Geometry: see drawing. Coordinates: mm, zero at the bounding-box minimum. A direction names the side the tool comes from. Give positions to 0.01 mm unless a question says otherwise; leave off trailing zeros. Order: outer loops, then holes, each group sorted by start corner. A loop starts at its lowest first (then second) coordinate and runs counter-clockwise, first axis right, second up. Notation, with made-up numbers: (13.5, 68.25) - (42.5, 68.25) arc R29 cw to (42.5, 100.25) - close; hole circle Ø6 at (-13.75, 35.25). An arc over 180 degrees is marked (long way). One line per item, written item: value.
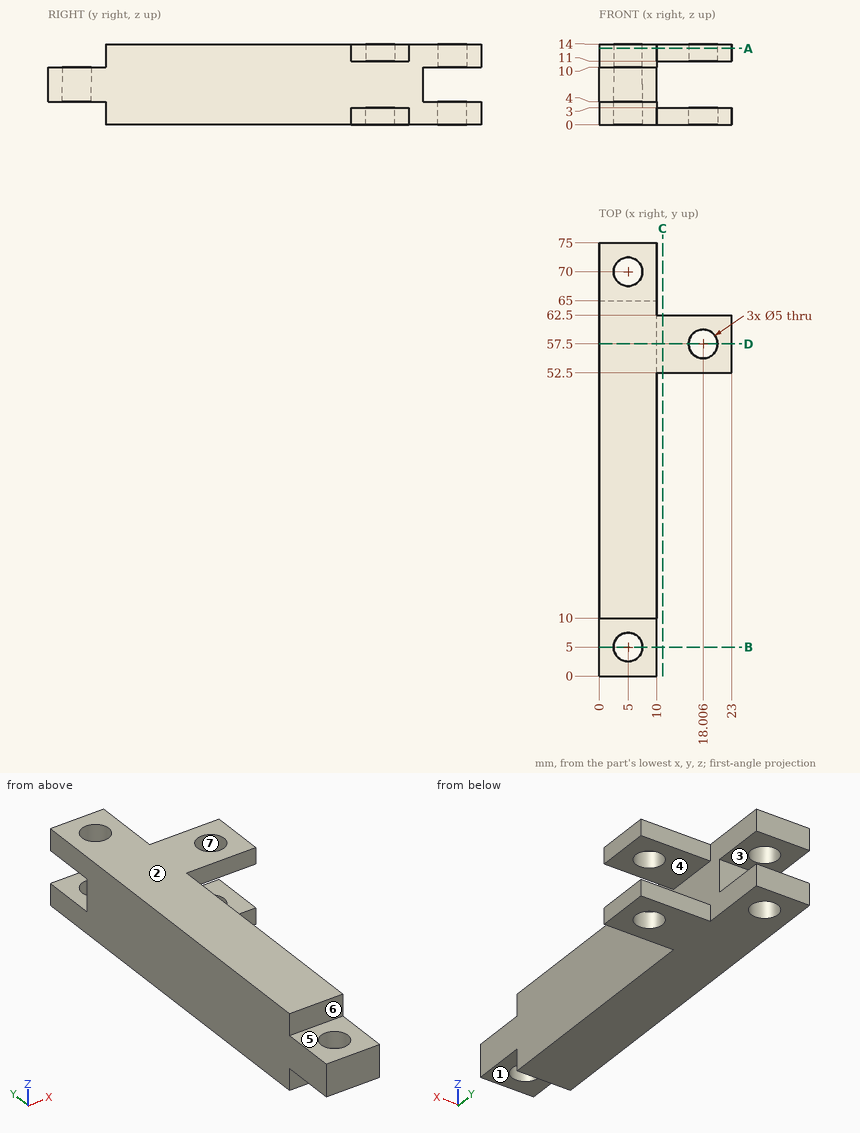
1) Set-up query: the marked faces 1, 2, 3 and 4. Return all of +Z, -Z, +X, -X, +Y, -Y with unobstructed straight access to the full face (end or side cutting, diameter ignored); none if empty.
Answers below:
face 1: -Z, +X, -X, -Y
face 2: +Z, +X, -X, +Y, -Y
face 3: +X, -X, +Y
face 4: +X, +Y, -Y
2) Mould query, pull axis Y, two halves, no side actions, for the marked faces 5, 6 and 7. Classes: released by +Y, released by -Y, zero draft, split by the parting line, or undercut.
Answers below:
face 5: zero draft
face 6: released by -Y
face 7: undercut
3) Section B-B, the plane y = 5. Return loops of the section in (x, z).
Answers below:
outline: (0, 4) - (2.5, 4) - (2.5, 10) - (0, 10) - close; (7.5, 4) - (10, 4) - (10, 10) - (7.5, 10) - close
4) Section A-A, the plane z = 13.25. Return loops of the section in (x, y) (1 decimal).
Answers below:
outline: (0, 10) - (10, 10) - (10, 52.5) - (23, 52.5) - (23, 62.5) - (10, 62.5) - (10, 75) - (0, 75) - close; hole circle Ø5 at (5, 70); hole circle Ø5 at (18, 57.5)
5) First-contact query: pin 1 (4 mm diameter, centred on x = 5, y = 70, fed in from +Z); pin 2 (6 mm diameter, centred on x = 5, y = 5, fed in from -Z); pin 3 (7 mm diameter, centred on y = 42, z = 6.5, fed in from +X); pin 4 (0.9 mm diameter, centred on x = 18, z = 2, fed in from -Y). Flat tips, straight axial feed; report the tip coordinate or a pass-through.
Answers below:
pin 1: through
pin 2: z = 4
pin 3: x = 10
pin 4: y = 52.5
6) Section C-C, the plane x = 11. Return loops of the section in (y, z).
Answers below:
outline: (52.5, 0) - (62.5, 0) - (62.5, 3) - (52.5, 3) - close; (52.5, 11) - (62.5, 11) - (62.5, 14) - (52.5, 14) - close
7) Material intervals for line 1 along X through (y, z) = (57, 8); line 2 along Y through (x, z) = (3.5, 4.25); line 3 along Y through (x, z) = (5, 1.55), sorted ascending.
Answers below:
line 1: 0 to 10
line 2: 0 to 3, 7 to 65
line 3: 10 to 67.5, 72.5 to 75
8) Section D-D, the plane y = 57.5. Return loops of the section in (x, z) (1 decimal).
Answers below:
outline: (0, 0) - (15.5, 0) - (15.5, 3) - (10, 3) - (10, 11) - (15.5, 11) - (15.5, 14) - (0, 14) - close; (20.5, 0) - (23, 0) - (23, 3) - (20.5, 3) - close; (20.5, 11) - (23, 11) - (23, 14) - (20.5, 14) - close
